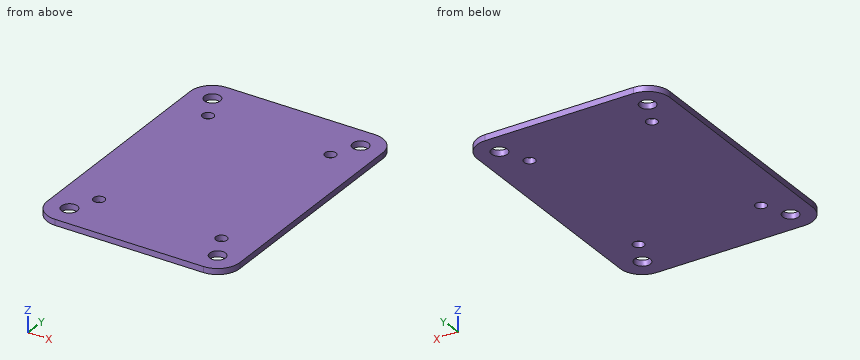
Solid Edge part; units mm, degrees
sketch "Sketch1" plane through (0, 0, 0) normal (0, 0, 1) x (1, 0, 0)
  line L0 (26, -36) -> (26, 36)
  line L1 (26, 36) -> (-26, 36)
  line L2 (-26, 36) -> (-26, -36)
  line L3 (-26, -36) -> (26, -36)
  circle A0 centre (20, 30) radius 2.15
  circle A1 centre (-20, -30) radius 2.15
  circle A2 centre (-20, 30) radius 2.15
  circle A3 centre (20, -30) radius 2.15
extrude "Protrusion1" add sketch "Sketch1" along normal blind 1.5875
fillet "Round_1" radius 6 4 edges at (-26, -36, 0.7937) (26, -36, 0.7937) (26, 36, 0.7937) (-26, 36, 0.7937)
sketch "Sketch2" plane through (0, 0, 1.5875) normal (0, 0, 1) x (1, 0, 0)
  circle A0 centre (16.47, 22.82) radius 1.5
  circle A1 centre (16.47, -22.9) radius 1.5
  circle A2 centre (-16.55, -22.9) radius 1.5
  circle A3 centre (-16.55, 22.82) radius 1.5
extrude "Cutout1" cut sketch "Sketch2" against normal up to next
properties material "Acrylic, high impact grade"
Design review of the part built by this model. Coordinates are the model's own, in mm. Round coordinates to 2 decimals unless told otherwise and drop trailing zeros. Order: outer loops, then holes, each group sorted by start corner. A loop starts at its lowest first (then second) coordinate and runs counter-clockwise, first axis right, second up.
1) For L1, parallel to Y at x = 16.47, z = 1; L2, parallel to Y at x = -20, z = 1.2; L3, parallel to X at y = -23.5, z = 1.1, list the stretches that pass through material, from the lowest coordinate up.
The answers:
L1: y = -36 to -24.4, -21.4 to 21.32, 24.32 to 36
L2: y = -36 to -32.15, -27.85 to 27.85, 32.15 to 36
L3: x = -26 to -17.92, -15.18 to 15.1, 17.84 to 26
2) Consider section A-A (y = 22.82). State the section outline as (x, z) points.
The answers:
outline: (-26, 0) - (-18.05, 0) - (-18.05, 1.59) - (-26, 1.59) - close; (-15.05, 0) - (14.97, 0) - (14.97, 1.59) - (-15.05, 1.59) - close; (17.97, 0) - (26, 0) - (26, 1.59) - (17.97, 1.59) - close
3) Consider section B-B (z = 0.8). Count the separate pieces of the cut face and the enclosed holes in it, plus the area to 3 significant figures.
The answers:
separate pieces: 1
enclosed holes: 8
area: 3,630 mm2
4) Consider section C-C (x = -16.55). State the section outline as (y, z) points.
The answers:
outline: (-36, 0) - (-24.4, 0) - (-24.4, 1.59) - (-36, 1.59) - close; (-21.4, 0) - (21.32, 0) - (21.32, 1.59) - (-21.4, 1.59) - close; (24.32, 0) - (36, 0) - (36, 1.59) - (24.32, 1.59) - close
